Design review of the part built by this model. Coordinates are the model's own, in mm. A direction names the side the tool comes from. Coordinates: 2 decimals unless noted, no trailing zeros. Loops run counter-clockwise (first coordinate to the right, second up) from the corner with the lowest first, then second, coordinate; pieces in that order, holes last. Notation, with made-up numbers: M 47.25,-3.75 L 89.25,-3.75 A37 cw 89.25,33.25 Z; hole C 30.5,-16 d10. An arc over 180 degrees is marked long. Write item = value, one per line. Start each with the question number.
Autodesk Fusion 360 part; units mm, degrees
sketch "Sketch1" plane through (0, 0, 0) normal (0, 0, 1) x (1, 0, 0)
  circle A0 centre (0, 0) radius 22.5
  circle A1 centre (0, 0) radius 19.35
  dimension "d1" = 45
  dimension "d2" = 38.7
extrude "Extrude1" add sketch "Sketch1" along normal blind 5 contours A1
extrude "Extrude2" add sketch "Sketch1" along normal blind 29
fillet "Fillet1" radius 1 1 edges at (-18.0405, 6.9973, 29)
fillet "Fillet2" radius 1 1 edges at (-20.9774, -8.1363, 0)
Q1. Clearance check with flat-ended pins moving along their axes: P1, Ø1, axis at x = -13, z = 6.5, coming from the +Y side; P2, Ø12, axis at x = -11, z = 14.5, coming from the +Y side; P3, Ø3, axis at x = -12, z = 26, coming from the -Y side. State where each tip first meets the part, or that it passes through.
Q2. For faces 1 (the face through (0, 0, 5)), 2 (the face through (0, 0, 0)), list the 3-axis set-ups (+Z, -Z, +X, -X, +Y, -Y) from which the entire face can be reached by the end or side of a thin tool; tool diameter is ignored.
Q3. Add section A-A on y = 0. State the section outline as (x, z) points, plus the area to 3 significant figures.
Q4. To check wall thickness, follow line 1 (Y direction, x = 0, z = 16.75); line 2 (Z direction, x = 2.5, y = 7.5); line 3 (X direction, y = 10.5, z = 23). State the ranges of each line that lie inside material, in increasing order. Write a range as from..to.
Q5. Add section D-D on z = 2. State the section outline as (x, y) points.
Q6. Mouldability with a two-part tool opening along X and no side actions: class faces 3 (the face through (-17, -12, 29)), 4 (the face through (-19.33, -0.85, 16.34)), 5 (the face through (10.382, 19.961, 14.804)) as released by +X, released by -X, zero draft, split by the parting line, or undercut.
Q7. Add section C-C on z = 6.25. State the section outline as (x, y) points.
Values follow:
q1.P1 = 18.71
q1.P2 = 21.94
q1.P3 = -19.9
q2.face_1 = +Z
q2.face_2 = -Z, +X, -X, +Y, -Y
q3.outline = M -22.5,1 A1 ccw -21.5,0 L 21.5,0 A1 ccw 22.5,1 L 22.5,29 L 20.35,29 A1 ccw 19.35,28 L 19.35,5 L -19.35,5 L -19.35,28 A1 ccw -20.35,29 L -22.5,29 Z
q3.area = 375 mm2
q4.line_1 = -22.5..-19.35, 19.35..22.5
q4.line_2 = 0..5
q4.line_3 = -19.9..-16.25, 16.25..19.9
q5.outline = C 0,0 d45
q6.face_3 = zero draft
q6.face_4 = undercut
q6.face_5 = split by the parting line
q7.outline = C 0,0 d45; hole C 0,0 d38.7
